Geometry check sheet. Reference: drawing and pictorial views, mm from the part's lowest x, y, z. A direction names the side the tool comes from. Give positions to 0.01 mm unless a question says otherwise; leave off trailing zeros. Order: outer loops, then holes, each group sorted by start corner. A loop starts at its lowest first (then second) coordinate and runs counter-clockwise, first axis right, second up. Notation, with made-up numbers: M -33,-40 L 2,-40 A26 cw 2,-12 Z; hole C 76.5,24 d1. An arc over 180 degrees is marked long. Answer as a JSON object with one key per item and string values. Group by question number.
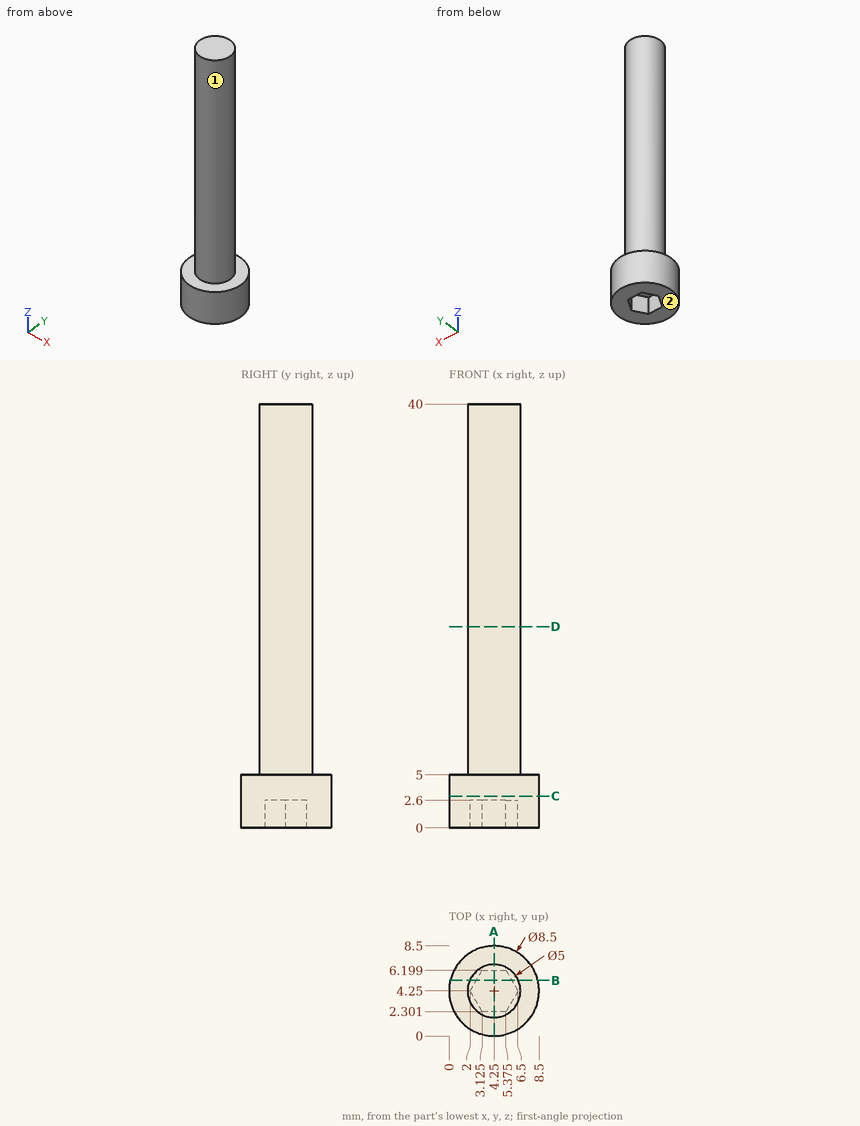
1. Cross-section at C-C (z = 3). Record the cut outline in (x, y).
2. Depth check by flat-ended pin: pin 1 (2 mm diameter, centred on x = 6.5, z = 14, fed in from -Y) (1 decimal); pin 2 (2.5 mm diameter, centred on x = 4, z = 1.5, fed in from +Y); pin 3 (3 mm diameter, centred on x = 4, z = 15.5, fed in from +Y); pin 4 (1.5 mm diameter, centred on x = 2.5, z = 27.5, fed in from +Y). Enter the tip coordinate at first touch or a pass-through.
3. Cross-section at A-A (x = 4.25). Record the cut outline in (y, z), and give its area (3 significant figures).
4. Thickness scan on line 1 along Z through (x, y) = (2.75, 7); line 2 along Z through (x, y) = (3.25, 4); line 3 along Y through (x, z) = (3, 2) (1 decimal). Record the ranges inside material, lowest first. Write a range as [from, to].
5. Access from +Z, -Z, +X, -X, +Y, -Y to the whole of each face (thin tool, end or side, straight path). Record for the marked faces 1 and 2.
6. Cross-section at B-B (y = 5.25). Record the cut outline in (x, z), and give its area (3 significant figures).
7. Cross-section at D-D (z = 19). Record the cut outline in (x, y).
Report:
{
 "1": {"outline": "C 4.25,4.25 d8.5"},
 "2": {"pin 1": "stops at y = 2.1", "pin 2": "stops at y = 8.5", "pin 3": "stops at y = 6.75", "pin 4": "stops at y = 6.54"},
 "3": {"outline": "M 0,0 L 2.3,0 L 2.3,2.6 L 6.2,2.6 L 6.2,0 L 8.5,0 L 8.5,5 L 6.75,5 L 6.75,40 L 1.75,40 L 1.75,5 L 0,5 Z", "area": "207 mm2"},
 "4": {"line 1": "z = [0, 5]", "line 2": "z = [2.6, 40]", "line 3": "y = [0.2, 2.5], [6, 8.3]"},
 "5": {"face 1": "+Z", "face 2": "-Z, +X, -X, +Y, -Y"},
 "6": {"outline": "M 0.12,0 L 2.58,0 L 2.58,2.6 L 5.92,2.6 L 5.92,0 L 8.38,0 L 8.38,5 L 6.54,5 L 6.54,40 L 1.96,40 L 1.96,5 L 0.12,5 Z", "area": "193 mm2"},
 "7": {"outline": "C 4.25,4.25 d5"}
}
